Geometry check sheet. Reference: the model listing, model coordinates, mm. Face numbers are marked on the shaded views. A direction names the side the tool comes from. Coordinates: 2 decimals unless noted, no trailing zeros. Write each loop counter-clockwise with the first axis right and the second up, starting at its lowest first coordinate (ties: lowest second). Pieces come first, ordered by that corner, then holes.
from build123d import *

# Parameters (mm, degrees)
SKETCH_1_R          = 4
EXTRUDE_1_DEPTH     = 45
SKETCH_2_R          = 4
CUT_EXTRUDE_1_DEPTH = 45


with BuildPart() as part:
    # 草图1 → 凸台-拉伸1 (new body)
    with BuildSketch(Plane(origin=(0, 0, 0), x_dir=(0, 0, -1), z_dir=(1, 0, 0))):
        with BuildLine():
            Line((-20, 15), (15, 15))
            ThreePointArc((15, 15), (18.535533906, 13.535533906), (20, 10))
            Line((20, 10), (20, -10))
            ThreePointArc((20, -10), (18.535533906, -13.535533906), (15, -15))
            Line((15, -15), (-20, -15))
            Line((-20, -15), (-20, -25))
            ThreePointArc((-20, -25), (-21.464466094, -28.535533906), (-25, -30))
            Line((-25, -30), (-45, -30))
            Line((-45, -30), (-45, 30))
            Line((-45, 30), (-25, 30))
            ThreePointArc((-25, 30), (-21.464466094, 28.535533906), (-20, 25))
            Line((-20, 25), (-20, 15))
        make_face()
        with Locations(Location((10, 0, 0), (0, 0, 180))):
            Circle(SKETCH_1_R, mode=Mode.SUBTRACT)
    extrude(amount=EXTRUDE_1_DEPTH)

    # 草图2 → 切除-拉伸1 (cut)
    with BuildSketch(Plane.XY.offset(45)):
        with Locations((22.5, 21)):
            Circle(SKETCH_2_R)
        with Locations(Location((22.5, -21, 0), (0, 0, 270))):
            Circle(SKETCH_2_R)
    extrude(amount=-CUT_EXTRUDE_1_DEPTH, mode=Mode.SUBTRACT)


solid = part.part
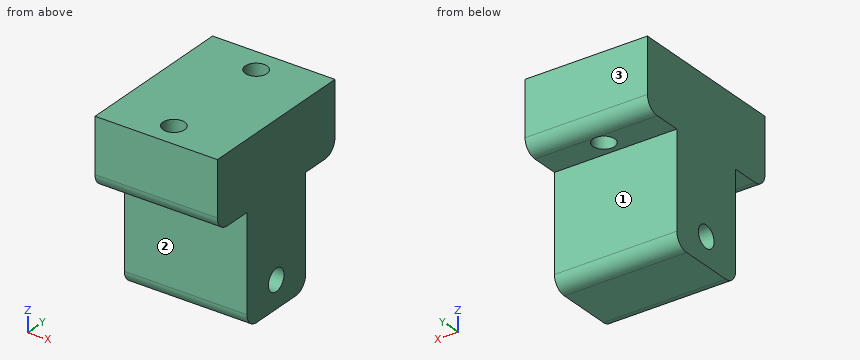
1. Sectioned sample at C-C, the plane x = 6. Record the boundary of the cut face in (y, z).
Computed values:
outline: (-30, 25) arc R5 ccw to (-25, 20) - (-15, 20) - (-15, -15) arc R5 ccw to (-10, -20) - (10, -20) arc R5 ccw to (15, -15) - (15, 20) - (25, 20) arc R5 ccw to (30, 25) - (30, 45) - (-30, 45) - close; hole circle Ø8 at (0, -10)
2. Access from +Z, -Z, +X, -X, +Y, -Y to the whole of each face (thin tool, end or side, straight path). Record for the marked faces 1, 2 and 3.
Computed values:
face 1: -Z, +X, -X, +Y
face 2: -Z, +X, -X, -Y
face 3: +Z, -Z, +X, -X, +Y
3. Gauge pin test, flat end, axial feed: pin 1 Ø5 at (x, y) = (31.5, -23) entering from -Z. Record the tip position at first contact, or that the pin passes through.
Computed values:
pin 1: stops at z = 20
4. Sectioned sample at D-D, the plane z = 29. Record the boundary of the cut face in (x, y), and give its area (3 significant figures).
Computed values:
outline: (0, -30) - (45, -30) - (45, 30) - (0, 30) - close; hole circle Ø8 at (22.5, -21); hole circle Ø8 at (22.5, 21)
area: 2,600 mm2
5. Sectioned sample at B-B, the plane z = -10. Record the boundary of the cut face in (x, y).
Computed values:
outline: (0, -15) - (45, -15) - (45, -4) - (0, -4) - close; (0, 4) - (45, 4) - (45, 15) - (0, 15) - close
6. Thickness scan on line 1 along Y through (x, z) = (18, -10); line 2 along X through (y, z) = (-21, 28); line 3 along Z through (x, y) = (33.5, -24). Record the ranges inside material, lowest first.
Computed values:
line 1: y = -15 to -4, 4 to 15
line 2: x = 0 to 18.5, 26.5 to 45
line 3: z = 20 to 45
7. Sectioned sample at A-A, the plane y = 0. Record the boundary of the cut face in (x, z), and give its area (4 significant figures).
Computed values:
outline: (0, -20) - (45, -20) - (45, -14) - (0, -14) - close; (0, -6) - (45, -6) - (45, 45) - (0, 45) - close
area: 2,565 mm2
